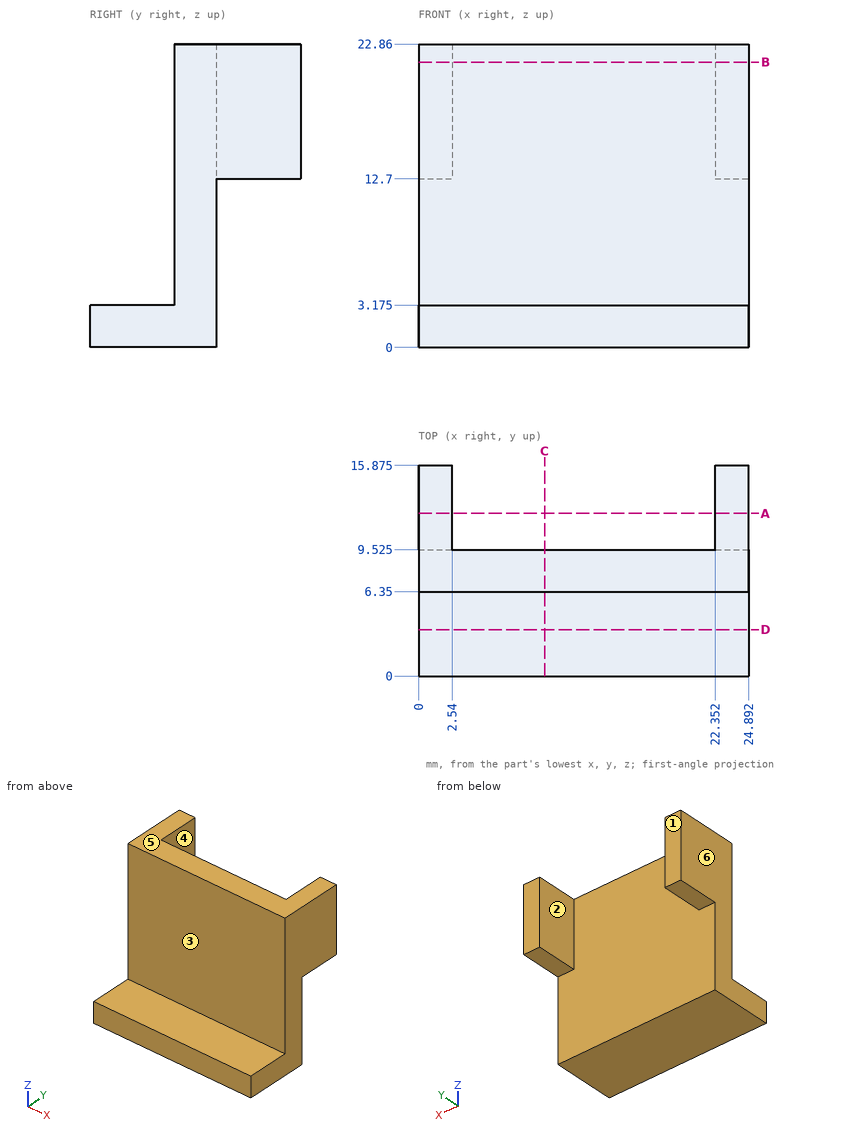
For this review, use the dimensioned drawing (mm, ordinates from the lowest corner) and the shaded views. A direction names the side the tool comes from. Give positions to 0.01 mm unless a question says otherwise; leave off trailing zeros. Order: outer loops, then holes, each group sorted by start corner. A loop starts at its lowest first (then second) coordinate and runs counter-clockwise, first axis right, second up. Notation, with made-up numbers: (64.25, 44.25) - (90.25, 44.25) arc R18 cw to (90.25, 52.25) - close; hole circle Ø5 at (9, 13). An arc over 180 degrees is marked (long way). Use CSV: the item, a comma, the result in double quotes. Start each with the question number.
Q1. We need section B-B, the plane z = 21.5. Write out the cut boundary in (x, y) (3 decimals).
Q2. The part is to be moulded in two halves that separate along X. For the marked faces 4, 5 and 6, say which applies: +X half, -X half, draft (parallel to the pull), parting line (faces both ways), or undercut.
Q3. Clearance check with flat-ended pins moving along their axes: pin 1 Ø4 at (x, z) = (6, 17) entering from +Y (3 decimals); pin 2 Ø0.8 at (x, y) = (24, 13.5) entering from -Z; pin 3 Ø1 at (y, z) = (11.5, 5) entering from +X (3 decimals). State where each tip first meets the part, or that it passes through.
Q4. We need section A-A, the plane y = 12.25. Write out the cut boundary in (x, z).
Q5. We need section D-D, the plane y = 3.5. Write out the cut boundary in (x, z) (3 decimals).
Q6. Tool access review of the marked faces 1, 2 and 3: name each direction out of +Z, -Z, +X, -X, +Y, -Y from which nothing blocks a thin tool from reaching the whole face with its end or side.
Q7. To check wall thickness, follow line 1 along X through (y, z) = (14.5, 21.5); line 2 along Y through (x, z) = (1.5, 3.25) (3 decimals); line 3 along Y through (x, z) = (18.5, 1.5) (3 decimals). State the ranges of each line that lie inside material, in increasing order. Write a range as [from, to].
Q8. We need section C-C, the plane x = 9.5. Write out the cut boundary in (y, z) (3 decimals).
Outcome:
1,outline,"(0, 6.35) - (24.892, 6.35) - (24.892, 15.875) - (22.352, 15.875) - (22.352, 9.525) - (2.54, 9.525) - (2.54, 15.875) - (0, 15.875) - close"
2,face 4,"undercut"
2,face 5,"draft"
2,face 6,"-X half"
3,pin 1,"stops at y = 9.525"
3,pin 2,"stops at z = 12.7"
3,pin 3,"passes through"
4,outline,"(0, 12.7) - (2.54, 12.7) - (2.54, 22.86) - (0, 22.86) - close; (22.35, 12.7) - (24.89, 12.7) - (24.89, 22.86) - (22.35, 22.86) - close"
5,outline,"(0, 0) - (24.892, 0) - (24.892, 3.175) - (0, 3.175) - close"
6,face 1,"+Z, -Z, +X, -X, +Y"
6,face 2,"+Z, -Z, +Y"
6,face 3,"+Z, +X, -X, -Y"
7,line 1,"x = [0, 2.54], [22.35, 24.89]"
7,line 2,"y = [6.35, 9.525]"
7,line 3,"y = [0, 9.525]"
8,outline,"(0, 0) - (9.525, 0) - (9.525, 22.86) - (6.35, 22.86) - (6.35, 3.175) - (0, 3.175) - close"
